Check sheet for the modelled part. Datum: model origin and axes. Units: mm. Face numbers are marked on the shaded views. Coordinates: 2 decimals unless noted, no trailing zeros. Loops run counter-clockwise (first coordinate to the right, second up) from the corner with the lowest first, then second, coordinate; pieces in that order, holes last.
Autodesk Inventor part; units mm, degrees
ref_plane "YZ Plane" through (0, 0, 0) normal (1, 0, 0) x (0, 1, 0)
ref_plane "XZ Plane" through (0, 0, 0) normal (0, 1, 0) x (-1, 0, 0)
ref_plane "XY Plane" through (0, 0, 0) normal (0, 0, 1) x (1, 0, 0)
sketch "Sketch1" plane through (0, 0, 0) normal (0, 0, 1) x (1, 0, 0)
  line L0 (0, 0) -> (25, 0)
  line L1 (25, 0) -> (25, 80)
  line L2 (25, 80) -> (0, 80)
  line L3 (0, 80) -> (0, 0)
  circle A0 centre (12.5, 11) radius 6.35
  dimension "d0" = 25
  dimension "d1" = 80
  dimension "d2" = 12.7
extrude "Extrusion1" add sketch "Sketch1" along normal blind 6
properties part number "Handle Connected"
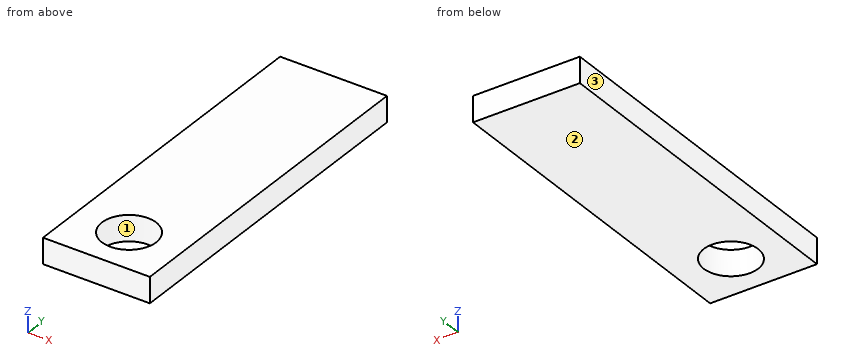
(1) Draft check along X on the marked faces 1, 2 and 3. Enter one of: pulls with the +X half, pulls with the -X half, needs draft (parallel to the pull), parting line crosses it, or undercut.
(2) Section check B-B, the plane x = 12.5. Enter the section's corners in (y, z).
(3) Section check C-C, the plane z = 1.7. Enter the section's corners in (x, y), plus the area to 3 significant figures.
(4) Gauge pin test, flat end, axial feed: P1, Ø7.5, axis at x = 12.5, y = 11, coming from the +Z side. Record the tip position at first contact, or that the pin passes through.
(5) Scan lines: line 1 along Y through (x, z) = (12.5, 3.9); line 2 along Y through (x, z) = (18, 2.5). Record each from-to range of solid material in increasing order.
(6) Section check A-A, the plane y = 11. Enter the section's corners in (x, z).
Determined:
1. face 1: undercut
1. face 2: needs draft
1. face 3: pulls with the -X half
2. outline: (0, 0) - (4.65, 0) - (4.65, 6) - (0, 6) - close; (17.35, 0) - (80, 0) - (80, 6) - (17.35, 6) - close
3. outline: (0, 0) - (25, 0) - (25, 80) - (0, 80) - close; hole circle Ø12.7 at (12.5, 11)
3. area: 1,870 mm2
4. P1: passes through
5. line 1: y = 0 to 4.65, 17.35 to 80
5. line 2: y = 0 to 7.83, 14.17 to 80
6. outline: (0, 0) - (6.15, 0) - (6.15, 6) - (0, 6) - close; (18.85, 0) - (25, 0) - (25, 6) - (18.85, 6) - close
